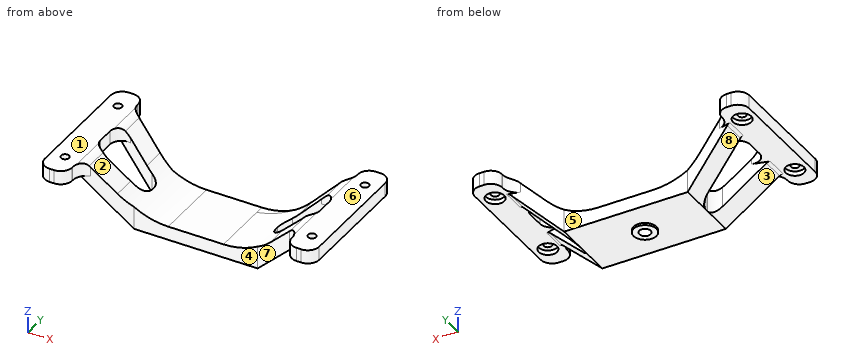
from build123d import *

# Parameters (mm, degrees)
EXTRUDE_1_DEPTH     = 60
SKETCH_2_R          = 1.75
CUT_EXTRUDE_1_DEPTH = 40
SKETCH_3_R          = 4
CUT_EXTRUDE_2_DEPTH = 2
SKETCH_4_R          = 2.5
CUT_EXTRUDE_3_DEPTH = 3
EXTRUDE_START       = 1
SKETCH_5_R          = 5
SKETCH_5_R_2        = 2.5
EXTRUDE_2_DEPTH     = 1
FILLET_1_R          = 5
FILLET_2_R          = 30
FILLET_4_R          = 2
FILLET_5_R          = 5
FILLET_6_R          = 6
FILLET_7_R          = 5


with BuildPart() as part:
    # 草图1 → 凸台-拉伸1 (new body)
    with BuildSketch(Plane(origin=(0, 0, 0), x_dir=(1, 0, 0), z_dir=(0, 1, 0))):
        Polygon((-24.514718626, 0), (24.514718626, 0), (45.514718626, -21), (60, -21), (60, -15), (48, -15), (27, 6), (-27, 6), (-48, -15), (-60, -15), (-60, -21), (-45.514718626, -21), align=None)
    extrude(amount=EXTRUDE_1_DEPTH)

    # 草图2 → 切除-拉伸1 (cut)
    with BuildSketch(Plane(origin=(0, 0, -6), x_dir=(-1, 0, 0), z_dir=(0, 0, -1))):
        with Locations((-54, 50)):
            Circle(SKETCH_2_R)
        with Locations((-54, 10)):
            Circle(SKETCH_2_R)
        with Locations((54, 10)):
            Circle(SKETCH_2_R)
        with Locations((54, 50)):
            Circle(SKETCH_2_R)
        Polygon((-48, 60), (-48, 50), (-27, 44.5), (27, 44.5), (48, 50), (48, 60), align=None)
        Polygon((48, 0), (48, 10), (27, 15.5), (-27, 15.5), (-48, 10), (-48, 0), align=None)
        Polygon((-48, 40), (-27, 34.5), (-27, 25.5), (-48, 20), align=None)
        Polygon((48, 20), (27, 25.5), (27, 34.5), (48, 40), align=None)
    extrude(amount=-CUT_EXTRUDE_1_DEPTH, mode=Mode.SUBTRACT)

    # 草图3 → 切除-拉伸2 (cut)
    with BuildSketch(Plane(origin=(0, 0, 15), x_dir=(-1, 0, 0), z_dir=(0, 0, -1))):
        with Locations((-54, 50)):
            Circle(SKETCH_3_R)
        with Locations(Location((-54, 10, 0), (0, 0, 180))):
            Circle(SKETCH_3_R)
        with Locations((54, 10)):
            Circle(SKETCH_3_R)
        with Locations(Location((54, 50, 0), (0, 0, 180))):
            Circle(SKETCH_3_R)
    extrude(amount=-CUT_EXTRUDE_2_DEPTH, mode=Mode.SUBTRACT)

    # 草图4 → 切除-拉伸3 (cut)
    with BuildSketch(Plane(origin=(0, 0, -6), x_dir=(-1, 0, 0), z_dir=(0, 0, -1))):
        with Locations((0, 30)):
            Circle(SKETCH_4_R)
    extrude(amount=-CUT_EXTRUDE_3_DEPTH, mode=Mode.SUBTRACT)

    # 草图5 → 凸台-拉伸2 (add)
    with BuildSketch(Plane(origin=(0, 0, -6), x_dir=(-1, 0, 0), z_dir=(0, 0, -1)).offset(EXTRUDE_START)):
        with Locations(Location((0, 30, 0), (0, 0, 180))):
            Circle(SKETCH_5_R)
        with Locations((0, 30)):
            Circle(SKETCH_5_R_2, mode=Mode.SUBTRACT)
    extrude(amount=-EXTRUDE_2_DEPTH)

    # 圆角1
    fillet_1_edges = [part.edges().sort_by_distance(p)[0] for p in [
        (60, 60, 18),
        (-60, 0, 18),
        (60, 0, 18),
        (-48, 0, 18),
        (48, 0, 18),
        (-60, 60, 18),
        (48, 60, 18),
        (-48, 60, 18),
    ]]
    fillet(fillet_1_edges, radius=FILLET_1_R)

    # 圆角2
    # the kernel refuses this fillet: 30 mm, written as the material it adds along each edge
    with BuildSketch(Plane(origin=(-24.514718626, -15.566017178, 0), x_dir=(-0.7071067811865465, 0, 0.7071067811865487), z_dir=(0, 1, 0))) as fillet_2_piece_1_section:
        with BuildLine():
            CenterArc((FILLET_2_R * 0.414213562373, FILLET_2_R), FILLET_2_R, 225, 45)
            Line((-FILLET_2_R * 0.292893218813, FILLET_2_R * 0.292893218813), (0, 0))
            Line((0, 0), (FILLET_2_R * 0.414213562373, 0))
        make_face()
    fillet_2_piece_1 = extrude(amount=91.132034356, mode=Mode.PRIVATE)
    fillet_2_piece_1 = split(fillet_2_piece_1, bisect_by=Plane(origin=(-29.494529343, 14.846670886, 5.3692292), z_dir=(-0.25335939183768474, 0.967372223380245, 0)), keep=Keep.TOP, mode=Mode.PRIVATE)
    fillet_2_piece_1 = split(fillet_2_piece_1, bisect_by=Plane(origin=(-31.945457725, 24.204761072, 5.3692292), z_dir=(0.2533593918376857, -0.9673722233802448, 0)), keep=Keep.TOP, mode=Mode.PRIVATE)
    add(fillet_2_piece_1)
    with BuildSketch(Plane(origin=(-24.514718626, 15.5, 0), x_dir=(-0.7071067811865465, 0, 0.7071067811865487), z_dir=(0, 1, 0))) as fillet_2_piece_2_section:
        with BuildLine():
            CenterArc((FILLET_2_R * 0.414213562373, FILLET_2_R), FILLET_2_R, 225, 45)
            Line((-FILLET_2_R * 0.292893218813, FILLET_2_R * 0.292893218813), (0, 0))
            Line((0, 0), (FILLET_2_R * 0.414213562373, 0))
        make_face()
    fillet_2_piece_2 = extrude(amount=29, mode=Mode.PRIVATE)
    fillet_2_piece_2 = split(fillet_2_piece_2, bisect_by=Plane(origin=(-27, 16.298150863, 0.780837191), z_dir=(1, 0, 0)), keep=Keep.TOP, mode=Mode.PRIVATE)
    add(fillet_2_piece_2)
    with BuildSketch(Plane(origin=(-24.514718626, -15.566017178, 0), x_dir=(-0.7071067811865465, 0, 0.7071067811865487), z_dir=(0, 1, 0))) as fillet_2_piece_3_section:
        with BuildLine():
            CenterArc((FILLET_2_R * 0.414213562373, FILLET_2_R), FILLET_2_R, 225, 45)
            Line((-FILLET_2_R * 0.292893218813, FILLET_2_R * 0.292893218813), (0, 0))
            Line((0, 0), (FILLET_2_R * 0.414213562373, 0))
        make_face()
    fillet_2_piece_3 = extrude(amount=91.132034356, mode=Mode.PRIVATE)
    fillet_2_piece_3 = split(fillet_2_piece_3, bisect_by=Plane(origin=(-29.759175244, 35.222641135, 4.528426502), z_dir=(0.25335939183768585, 0.9673722233802448, 0)), keep=Keep.TOP, mode=Mode.PRIVATE)
    fillet_2_piece_3 = split(fillet_2_piece_3, bisect_by=Plane(origin=(-27.308246862, 44.580731321, 4.528426502), z_dir=(-0.2533593918376847, -0.967372223380245, 0)), keep=Keep.TOP, mode=Mode.PRIVATE)
    add(fillet_2_piece_3)
    with BuildSketch(Plane(origin=(24.514718626, -15.566017178, 0), x_dir=(0.7071067811865461, 0, 0.7071067811865488), z_dir=(0, 1, 0))) as fillet_2_piece_4_section:
        with BuildLine():
            CenterArc((FILLET_2_R * 0.414213562373, -FILLET_2_R), FILLET_2_R, 90, 45)
            Line((-FILLET_2_R * 0.292893218813, -FILLET_2_R * 0.292893218813), (0, 0))
            Line((0, 0), (FILLET_2_R * 0.414213562373, 0))
        make_face()
    fillet_2_piece_4 = extrude(amount=91.132034356, mode=Mode.PRIVATE)
    fillet_2_piece_4 = split(fillet_2_piece_4, bisect_by=Plane(origin=(29.494529343, 14.846670886, 5.3692292), z_dir=(0.25335939183768474, 0.967372223380245, 0)), keep=Keep.TOP, mode=Mode.PRIVATE)
    fillet_2_piece_4 = split(fillet_2_piece_4, bisect_by=Plane(origin=(31.945457725, 24.204761072, 5.3692292), z_dir=(-0.25335939183768474, -0.967372223380245, 0)), keep=Keep.TOP, mode=Mode.PRIVATE)
    add(fillet_2_piece_4)
    with BuildSketch(Plane(origin=(24.514718626, 15.5, 0), x_dir=(0.7071067811865461, 0, 0.7071067811865488), z_dir=(0, 1, 0))) as fillet_2_piece_5_section:
        with BuildLine():
            CenterArc((FILLET_2_R * 0.414213562373, -FILLET_2_R), FILLET_2_R, 90, 45)
            Line((-FILLET_2_R * 0.292893218813, -FILLET_2_R * 0.292893218813), (0, 0))
            Line((0, 0), (FILLET_2_R * 0.414213562373, 0))
        make_face()
    fillet_2_piece_5 = extrude(amount=60.066017178, mode=Mode.PRIVATE)
    fillet_2_piece_5 = split(fillet_2_piece_5, bisect_by=Plane(origin=(27, 16.298150863, 0.780837191), z_dir=(-1, 0, 0)), keep=Keep.TOP, mode=Mode.PRIVATE)
    fillet_2_piece_5 = split(fillet_2_piece_5, bisect_by=Plane(origin=(14.384200648, 41.195862074, 0.780837191), z_dir=(0.2533593918376847, -0.967372223380245, 0)), keep=Keep.TOP, mode=Mode.PRIVATE)
    add(fillet_2_piece_5)
    with BuildSketch(Plane(origin=(24.514718626, -15.566017178, 0), x_dir=(0.7071067811865461, 0, 0.7071067811865488), z_dir=(0, 1, 0))) as fillet_2_piece_6_section:
        with BuildLine():
            CenterArc((FILLET_2_R * 0.414213562373, -FILLET_2_R), FILLET_2_R, 90, 45)
            Line((-FILLET_2_R * 0.292893218813, -FILLET_2_R * 0.292893218813), (0, 0))
            Line((0, 0), (FILLET_2_R * 0.414213562373, 0))
        make_face()
    fillet_2_piece_6 = extrude(amount=91.132034356, mode=Mode.PRIVATE)
    fillet_2_piece_6 = split(fillet_2_piece_6, bisect_by=Plane(origin=(29.759175244, 35.222641135, 4.528426502), z_dir=(-0.2533593918376849, 0.967372223380245, 0)), keep=Keep.TOP, mode=Mode.PRIVATE)
    fillet_2_piece_6 = split(fillet_2_piece_6, bisect_by=Plane(origin=(27.308246862, 44.580731321, 4.528426502), z_dir=(0.2533593918376847, -0.967372223380245, 0)), keep=Keep.TOP, mode=Mode.PRIVATE)
    add(fillet_2_piece_6)
    with BuildSketch(Plane(origin=(24.514718626, -15.566017178, 0), x_dir=(0.7071067811865461, 0, 0.7071067811865488), z_dir=(0, 1, 0))) as fillet_2_piece_7_section:
        with BuildLine():
            CenterArc((FILLET_2_R * 0.414213562373, -FILLET_2_R), FILLET_2_R, 90, 45)
            Line((-FILLET_2_R * 0.292893218813, -FILLET_2_R * 0.292893218813), (0, 0))
            Line((0, 0), (FILLET_2_R * 0.414213562373, 0))
        make_face()
    fillet_2_piece_7 = extrude(amount=60.066017178, mode=Mode.PRIVATE)
    fillet_2_piece_7 = split(fillet_2_piece_7, bisect_by=Plane(origin=(21.100650835, 42.954932361, 0.780837191), z_dir=(-0.2533593918376847, 0.967372223380245, 0)), keep=Keep.TOP, mode=Mode.PRIVATE)
    add(fillet_2_piece_7)

    # 圆角4
    fillet_4_edges = [part.edges().sort_by_distance(p)[0] for p in [
        (-48, 45, 15),
        (-48, 15, 15),
        (48, 45, 15),
        (48, 15, 15),
    ]]
    fillet(fillet_4_edges, radius=FILLET_4_R)

    # 圆角5
    fillet_5_edges = [part.edges().sort_by_distance(p)[0] for p in [
        (-45.514718626, 44.349092973, 21),
        (-45.514718626, 15.650907027, 21),
        (45.514718626, 44.349092973, 21),
        (45.514718626, 15.650907027, 21),
    ]]
    fillet(fillet_5_edges, radius=FILLET_5_R)

    # 圆角6
    fillet_6_edges = [part.edges().sort_by_distance(p)[0] for p in [
        (48, 50, 18),
        (-48, 50, 18),
        (-48, 10, 18),
        (48, 10, 18),
    ]]
    fillet(fillet_6_edges, radius=FILLET_6_R)

    # 圆角7
    fillet_7_edges = [part.edges().sort_by_distance(p)[0] for p in [
        (-48, 20, 18),
        (-48, 40, 18),
        (48, 40, 18),
        (48, 20, 18),
        (27, 25.5, -1.015774599),
        (27, 34.5, -1.015774599),
        (-27, 25.5, -1.015774599),
        (-27, 34.5, -1.015774599),
    ]]
    fillet(fillet_7_edges, radius=FILLET_7_R)


solid = part.part
Design review of the part built by this model. Coordinates are the model's own, in mm. Face numbers are marked on the shaded views. A direction names the side the tool comes from. Round coordinates to 2 decimals unless told otherwise and drop trailing zeros. Write each loop counter-clockwise with the first axis right and the second up, starting at its lowest first coordinate (ties: lowest second). Pieces come first, ordered by that corner, then holes. Notation, with made-up numbers: (0, 32.5) - (13, 32.5) arc R24 cw to (13, 67.5) - close; hole circle Ø1 at (-25, 85.5). An arc over 180 degrees is marked (long way). Use a Markdown table: item, result. Add a question column.
1. We need section C-C (x = 19). State the section outline as (y, z) points.
2. Mouldability with a two-part tool opening along X and no side actions: class the marked faces 6, 7 and 8 as +X half, -X half, draft (parallel to the pull), parting line (faces both ways), or undercut.
3. We need section A-A (x = 37.5). State the section outline as (y, z) points, then the cut area to 3 significant figures.
4. We need section B-B (x = 0). State the section outline as (y, z) points.
5. Wall thickness on probe 1 along Y at (x, z) = (-54, 16.6); probe 2 along Y at (x, z) = (54, 18.9); probe 3 along Z at (x, y) = (53, 29.5): over which ranges is each line inside the solid? List them lowest first.
6. We need section D-D (x = -24.5). State the section outline as (y, z) points, then the cut area to 3 significant figures.
7. Clearance check with flat-ended pins moving along their axes: pin 1 (10.5 mm diameter, centred on x = -54, y = 10, fed in from -Z); pin 2 (1.5 mm diameter, centred on x = 45, y = 38.5, fed in from +Z); pin 3 (9 mm diameter, centred on x = -52.5, y = 51, fed in from -Z). State where each tip first meets the part, or that it passes through.
8. For the marked faces 1, 2, 3, 4 and 5, list the 3-axis set-ups (+Z, -Z, +X, -X, +Y, -Y) from which the entire face can be reached by the end or side of a thin tool; tool diameter is ignored.
Output:
| question | item | result |
|---|---|---|
| 1 | outline | (15.5, -6) - (44.5, -6) - (44.5, 0.81) - (15.5, 0.81) - close |
| 2 | face 6 | draft |
| 2 | face 7 | undercut |
| 2 | face 8 | -X half |
| 3 | outline | (12.75, 4.5) - (22.75, 4.5) - (22.75, 12.99) - (12.75, 12.99) - close; (37.25, 4.5) - (47.25, 4.5) - (47.25, 12.99) - (37.25, 12.99) - close |
| 3 | area | 170 mm2 |
| 4 | outline | (15.5, -6) - (25, -6) - (25, -7) - (27.5, -7) - (27.5, -3) - (32.5, -3) - (32.5, -7) - (35, -7) - (35, -6) - (44.5, -6) - (44.5, 0) - (15.5, 0) - close |
| 5 | probe 1 | y = 0 to 6, 14 to 46, 54 to 60 |
| 5 | probe 2 | y = 0 to 8.25, 11.75 to 48.25, 51.75 to 60 |
| 5 | probe 3 | z = 15 to 21 |
| 6 | outline | (15.5, -6) - (44.5, -6) - (44.5, 2.69) - (15.5, 2.69) - close |
| 6 | area | 252 mm2 |
| 7 | pin 1 | stops at z = 15 |
| 7 | pin 2 | stops at z = 20.65 |
| 7 | pin 3 | stops at z = 14.87 |
| 8 | face 1 | +Z, +X, -X, +Y, -Y |
| 8 | face 2 | +Z, +Y, -Y |
| 8 | face 3 | -Z, -X, +Y, -Y |
| 8 | face 4 | +Z, -Z, -Y |
| 8 | face 5 | +Z, -Z, +Y |
